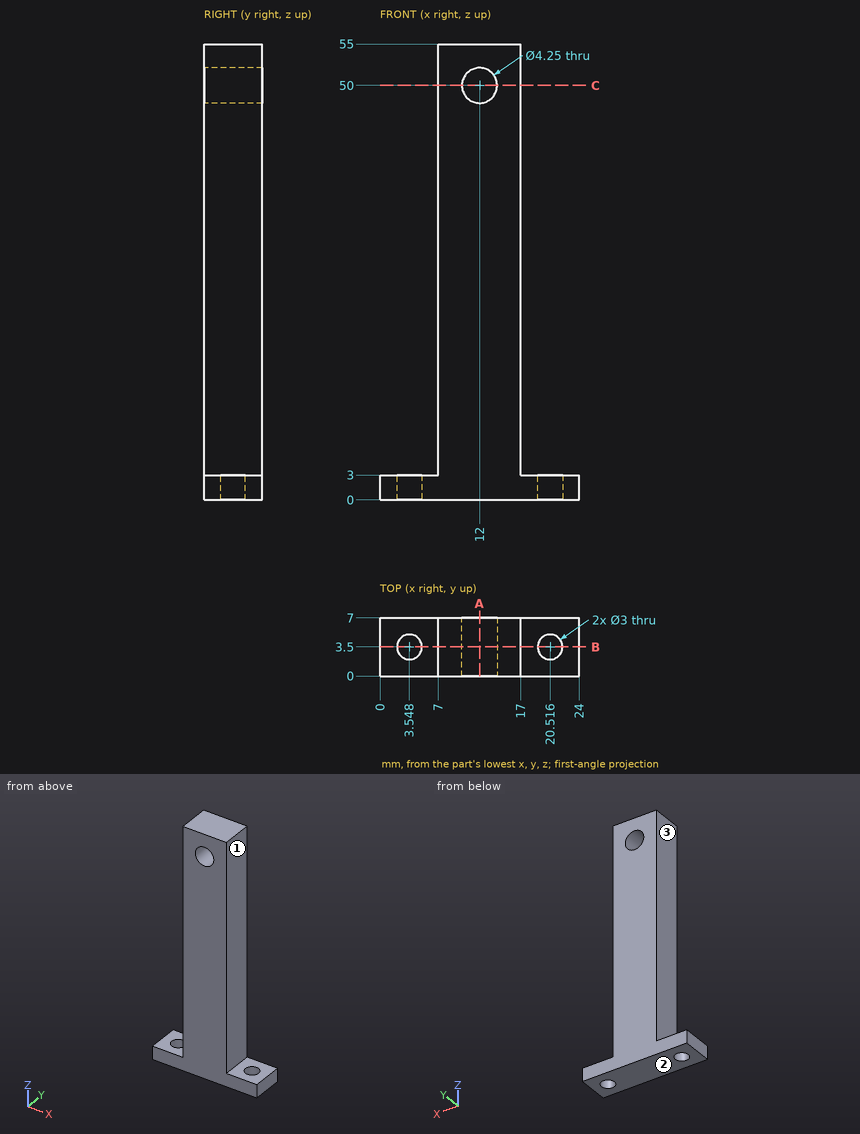
Answer from the drawing. Dimensions are ordinates in mm from the lowest x, y and z of the part. A direction names the side the tool comes from. Round coordinates to 2 decimals unless told otherwise and drop trailing zeros. Loops run counter-clockwise (first coordinate to the right, second up) from the corner with the lowest first, then second, coordinate; pieces in that order, holes last.
Q1. Section B-B on y = 3.5 is taken. Give the number of separate pieces and of enclosed holes in the cut face, and give its area (3 significant figures).
Q2. Section C-C on z = 50 is taken. Write down the section's boundary in (x, y) (1 decimal).
Q3. Which of the six approach directions +Z, -Z, +X, -X, +Y, -Y give full straight-line access (tool end or side, diameter ignored) to the marked faces 1, 2 and 3?
Q4. Each of these flat-tipped pins is pushed along its axis until it touches: pin 1 (2 mm diameter, centred on x = 22, y = 5, fed in from +Z); pin 2 (4 mm diameter, centred on y = 3.5, z = 30, fed in from +X); pin 3 (1 mm diameter, centred on y = 2.5, z = 34, fed in from -X); pin 4 (6 mm diameter, centred on x = 3.5, z = 14, fed in from +Y). Where does it stop, or does it pass through?
Q5. Consider probe 1 along Z at (x, y) = (12, 3.25) (1 decimal); probe 2 along X at (y, z) = (2.75, 50) (1 decimal); probe 3 along Z at (x, y) = (2, 5.25). Determine where each line is inside the solid, lowest interval first.
Q6. Section A-A on x = 12 is taken. Write down the section's boundary in (y, z) (1 decimal), and give its area (3 significant figures).
Output:
1. separate pieces: 3
1. enclosed holes: 1
1. area: 560 mm2
2. outline: (7, 0) - (9.9, 0) - (9.9, 7) - (7, 7) - close; (14.1, 0) - (17, 0) - (17, 7) - (14.1, 7) - close
3. face 1: +Z, +X, +Y, -Y
3. face 2: -Z, +X, -X, +Y, -Y
3. face 3: +Z, -X, +Y, -Y
4. pin 1: stops at z = 3
4. pin 2: stops at x = 17
4. pin 3: stops at x = 7
4. pin 4: passes through
5. probe 1: z = 0 to 47.9, 52.1 to 55
5. probe 2: x = 7 to 9.9, 14.1 to 17
5. probe 3: z = 0 to 3
6. outline: (0, 0) - (7, 0) - (7, 47.9) - (0, 47.9) - close; (0, 52.1) - (7, 52.1) - (7, 55) - (0, 55) - close
6. area: 355 mm2
